Geometry: final body of the model. Coordinates: model frame, mm. Give positions to 0.01 mm unless a question says otherwise; leave off trailing zeros. Order: outer loops, then holes, each group sorted by start corner. A loop starts at its lowest first (then second) coordinate and runs counter-clockwise, first axis right, second up. Notation, with made-up numbers: (-37, -20) -> (15, -20) arc R24 ccw to (15, 19) -> close; hole circle Ø3 at (76.25, 32.25). An arc over 180 degrees is marked (long way). Answer in a Markdown table with one row per item. Add a question column.
Q1. Contact query for flat-ended pins moving along their axis: P1, Ø1, axis at x = -2, z = 4, coming from the +Y side; P2, Ø1, axis at y = 1.5, z = 10, coming from the +X side; P3, Ø2, axis at x = -2, z = 5.5, coming from the +Y side. Output: stop coordinate, or through.
Q2. Cut plane C-C on z = 1.25. Return the cut outline in (x, y), and give its area (3 significant figures).
Q3. Pull-direction query (X, two-part tool) for faces 1 (the face through (-3, 0, 6)), 2 (the face through (-1.825, -1.4, 7.81)), 3 (the face through (0, -2, 2)), 4 (the face through (1, -2, 0)); classes: +X half, -X half, draft (parallel to the pull), parting line (faces both ways), or undercut.
Q4. Cut plane A-A on y = 0. Return the cut outline in (x, z), and give its area (3 significant figures).
Q5. Line query: line 1 along Y through (x, z) = (0, 7.75); line 2 along Y through (x, z) = (1.25, 3.25); line 3 along X through (y, z) = (1.7, 9.5). Output: solid intervals per line, ascending. Write a range as from..to.
Q6. Cut plane D-D on z = 5.25. Return the cut outline in (x, y).
from build123d import *

# Parameters (mm, degrees)
ESBO_O1_R                = 3
RESSALTO_EXTRUS_O1_DEPTH = 12
ESBO_O2_R                = 2.3
CORTE_EXTRUS_O1_DEPTH    = 8.5
CORTE_EXTRUS_O2_REACH    = 11.5
ESBO_O3_R                = 2


with BuildPart() as part:
    # Esboço1 → Ressalto-extrusão1 (new body)
    with BuildSketch(Plane.XY):
        Circle(ESBO_O1_R)
    extrude(amount=RESSALTO_EXTRUS_O1_DEPTH)

    # Esboço2 → Corte-extrusão1 (cut)
    with BuildSketch(Plane.XY.offset(12)):
        Circle(ESBO_O2_R)
    extrude(amount=-CORTE_EXTRUS_O1_DEPTH, mode=Mode.SUBTRACT)

    # Esboço3 → Corte-extrusão2 (cut, up to next)
    with BuildSketch(Plane.XY.offset(3.5), mode=Mode.PRIVATE) as corte_extrus_o2_sk1:
        Circle(ESBO_O3_R)
    corte_extrus_o2_tool1 = extrude(corte_extrus_o2_sk1.sketch, amount=-CORTE_EXTRUS_O2_REACH, mode=Mode.PRIVATE) & part.part
    add(corte_extrus_o2_tool1.solids().sort_by_distance((0, 0, 3.5))[0], mode=Mode.SUBTRACT)


solid = part.part
Completed:
| question | item | result |
|---|---|---|
| 1 | P1 | stops at y = 2.6 |
| 1 | P2 | stops at x = 2.83 |
| 1 | P3 | stops at y = 2.83 |
| 2 | outline | circle Ø6 at (0, 0); hole circle Ø4 at (0, 0) |
| 2 | area | 15.7 mm² |
| 3 | face 1 | parting line |
| 3 | face 2 | undercut |
| 3 | face 3 | undercut |
| 3 | face 4 | draft |
| 4 | outline | (-3, 0) -> (-2, 0) -> (-2, 3.5) -> (-2.3, 3.5) -> (-2.3, 12) -> (-3, 12) -> close; (2, 0) -> (3, 0) -> (3, 12) -> (2.3, 12) -> (2.3, 3.5) -> (2, 3.5) -> close |
| 4 | area | 18.9 mm² |
| 5 | line 1 | y = -3..-2.3, 2.3..3 |
| 5 | line 2 | y = -2.73..-1.56, 1.56..2.73 |
| 5 | line 3 | x = -2.47..-1.55, 1.55..2.47 |
| 6 | outline | circle Ø6 at (0, 0); hole circle Ø4.6 at (0, 0) |
